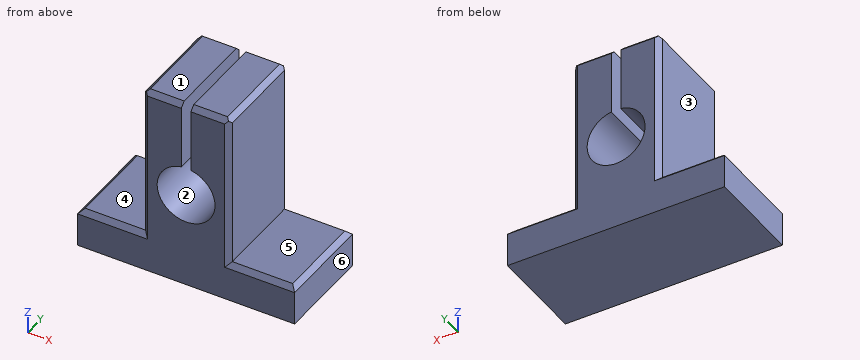
```python
from build123d import *

# Parameters (mm, degrees)
F1_DEPTH = 20
F2_SIZE  = 1
F3_SIZE  = 1
F4_SIZE  = 1


with BuildPart() as f1:
    # F0 (on Front) → F1 (new body)
    with BuildSketch(Plane.XZ):
        with BuildLine():
            Line((-9, -12), (-22.5, -12))
            Line((-22.5, -12), (-22.5, -20))
            Line((-22.5, -20), (22.5, -20))
            Line((22.5, -20), (22.5, -12))
            Line((22.5, -12), (9, -12))
            Line((9, -12), (9, 20))
            Line((9, 20), (1, 20))
            Line((1, 20), (1, 5.91608))
            ThreePointArc((1, 5.91608), (0, -6), (-1, 5.91608))
            Line((-1, 5.91608), (-1, 20))
            Line((-1, 20), (-9, 20))
            Line((-9, 20), (-9, -12))
        make_face()
    extrude(amount=F1_DEPTH)

    # F2
    f2_edges = [f1.edges().sort_by_distance(p)[0] for p in [
        (-5, -20, 20),
        (-5, 0, 20),
        (5, 0, 20),
        (5, -20, 20),
        (9, -10, 20),
        (-9, -10, 20),
    ]]
    chamfer(f2_edges, length=F2_SIZE)

    # F3
    f3_edges = [f1.edges().sort_by_distance(p)[0] for p in [
        (15.75, 0, -12),
        (15.75, -20, -12),
        (22.5, -10, -12),
        (-15.75, -20, -12),
        (-22.5, -10, -12),
        (-15.75, 0, -12),
    ]]
    chamfer(f3_edges, length=F3_SIZE)

    # F4
    f4_edges = [f1.edges().sort_by_distance(p)[0] for p in [
        (9, 0, 3.5),
        (-9, 0, 3.5),
        (9, -20, 3.5),
        (-9, -20, 3.5),
    ]]
    chamfer(f4_edges, length=F4_SIZE)


solid = f1.part
```
Geometry check sheet. Reference: the model listing, model coordinates, mm. Face numbers are marked on the shaded views. A direction names the side the tool comes from. Coordinates: 2 decimals unless noted, no trailing zeros. Order: outer loops, then holes, each group sorted by start corner. A loop starts at its lowest first (then second) coordinate and runs counter-clockwise, first axis right, second up. Notation, with made-up numbers: (24, 48) - (52, 48) arc R20 ccw to (52, 60) - close; hole circle Ø11 at (57, 29.5). An arc over 180 degrees is marked (long way). Answer in a Markdown table with one row per item. Add a question column.
1. Section check B-B (x = 4.5). Enter the section's corners in (y, z), plus the area to 3 significant figures.
2. Gauge pin test, flat ends, axial feed: pin 1 Ø7 at (x, z) = (0, 0) entering from +Y; pin 2 Ø1.5 at (x, z) = (-9.5, -11) entering from +Y; pin 3 Ø8 at (y, z) = (-11.5, 8) entering from +X; pin 4 Ø8 at (x, y) = (16, -14.5) entering from +Z. Record the tip position at first contact, or that the pin passes through.
3. Draft check along X on the marked faces 1, 2 and 3. Enter one of: +X half, -X half, draft (parallel to the pull), parting line (faces both ways), or undercut.
4. Section check A-A (z = 0). Enter the section's corners in (x, y), plus the area to 3 significant figures.
5. Material ranges on L1, parallel to X at y = -12.75, z = 0; L2, parallel to X at y = -9, z = 9.5; L3, parallel to Z at x = -19.5, y = -5, recorded low to high. Write a range as [from, to].
6. Access from +Z, -Z, +X, -X, +Y, -Y to the whole of each face (thin tool, end or side, straight path). Record for the marked faces 4, 5 and 6.
7. Section check D-D (y = -15.75). Enter the section's corners in (x, z).
8. Section check C-C (z = -7). Enter the section's corners in (x, y).
Data:
| question | item | result |
|---|---|---|
| 1 | outline | (-20, -20) - (0, -20) - (0, -3.97) - (-20, -3.97) - close; (-20, 3.97) - (0, 3.97) - (0, 19) - (-1, 20) - (-19, 20) - (-20, 19) - close |
| 1 | area | 640 mm² |
| 2 | pin 1 | passes through |
| 2 | pin 2 | stops at y = -0.75 |
| 2 | pin 3 | stops at x = 9 |
| 2 | pin 4 | stops at z = -12 |
| 3 | face 1 | draft |
| 3 | face 2 | undercut |
| 3 | face 3 | -X half |
| 4 | outline | (-9, -19) - (-8, -20) - (-6, -20) - (-6, 0) - (-8, 0) - (-9, -1) - close; (6, -20) - (8, -20) - (9, -19) - (9, -1) - (8, 0) - (6, 0) - close |
| 4 | area | 118 mm² |
| 5 | L1 | x = [-9, -6], [6, 9] |
| 5 | L2 | x = [-9, -1], [1, 9] |
| 5 | L3 | z = [-20, -12] |
| 6 | face 4 | +Z, -X, +Y, -Y |
| 6 | face 5 | +Z, +X, +Y, -Y |
| 6 | face 6 | +Z, -Z, +X, +Y, -Y |
| 7 | outline | (-22.5, -20) - (22.5, -20) - (22.5, -13) - (21.5, -12) - (9, -12) - (9, 19) - (8, 20) - (1, 20) - (1, 5.92) arc R6 cw (long way) to (-1, 5.92) - (-1, 20) - (-8, 20) - (-9, 19) - (-9, -12) - (-21.5, -12) - (-22.5, -13) - close |
| 8 | outline | (-9, -19) - (-8, -20) - (8, -20) - (9, -19) - (9, -1) - (8, 0) - (-8, 0) - (-9, -1) - close |
